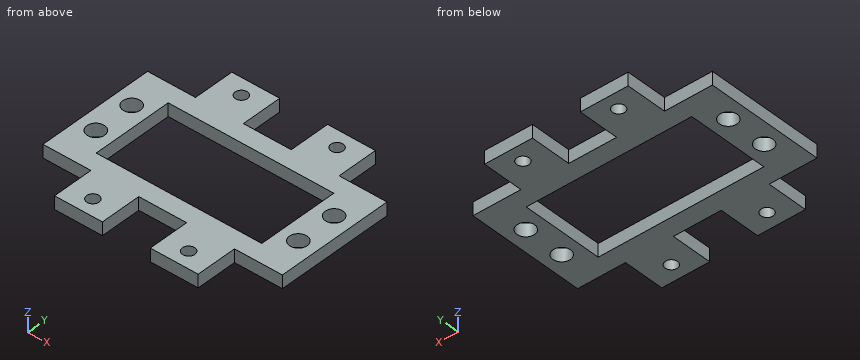
```python
from build123d import *

# Parameters (mm, degrees)
SKETCH2_R           = 2.15
SKETCH2_R_2         = 1.5
BOSS_EXTRUDE1_DEPTH = 3.175


with BuildPart() as part:
    # Sketch2 → Boss-Extrude1 (new body)
    with BuildSketch(Plane.XY):
        Polygon((23.312, 14.4), (29.14, 14.4), (29.14, 9.91), (8.98, 9.91), (8.98, 0), (0, 0), (0, 14.4), (11.656, 14.4), (11.656, 24.4), (23.312, 24.4), align=None)
        with Locations((4.49, 4.935)):
            Circle(SKETCH2_R, mode=Mode.SUBTRACT)
        with Locations((17.484, 20.43125)):
            Circle(SKETCH2_R_2, mode=Mode.SUBTRACT)
    boss_extrude1 = extrude(amount=BOSS_EXTRUDE1_DEPTH)

    # Mirror8: Boss-Extrude1 across plane
    add(boss_extrude1.mirror(Plane(origin=(8.98, 0, 3.175), x_dir=(0, 0, 1), z_dir=(0, 1, 0))))

    # Mirror10: part across plane


with BuildPart() as part_1:
    add(part.part)
    add(part.part.mirror(Plane(origin=(29.14, 9.91, 3.175), x_dir=(0, 0, 1), z_dir=(-1, 0, 0))))


solid = part_1.part
```
Read the model definition and answer for the solid it produces. Units are mm, in the model's axes. Round coordinates to 2 decimals unless told otherwise and drop trailing zeros. Write each loop counter-clockwise with the first axis right and the second up, starting at its lowest first coordinate (ties: lowest second). Pieces come first, ordered by that corner, then holes. Notation, with made-up numbers: (-4, 32) - (35, 32) arc R16 ccw to (35, 62) - close; hole circle Ø10 at (46.5, 42.25). An arc over 180 degrees is marked (long way). Use CSV: the item, a comma, the result in double quotes.
Q1. Find section C-C, the plane x = 53.79. Write down the section's boundary in (y, z) (3 decimals).
Values:
outline,"(-14.4, 0) - (-7.085, 0) - (-7.085, 3.175) - (-14.4, 3.175) - close; (-2.785, 0) - (2.785, 0) - (2.785, 3.175) - (-2.785, 3.175) - close; (7.085, 0) - (14.4, 0) - (14.4, 3.175) - (7.085, 3.175) - close"
Q2. Straight lines are drawn through the part: line 1 along X through (y, z) = (5, 0.45); line 2 along Y through (x, z) = (4.49, 1.6) (3 decimals); line 3 along Y through (x, z) = (37.5, 2). For each, find the intervals that lie inside material, in ascending order.
Values:
line 1,"x = 0 to 2.34, 6.64 to 8.98, 49.3 to 51.64, 55.94 to 58.28"
line 2,"y = -14.4 to -7.085, -2.785 to 2.785, 7.085 to 14.4"
line 3,"y = -24.4 to -9.91, 9.91 to 24.4"
Q3. Each of these flat-tipped pins is pushed along its axis until it touches: pin 1 Ø1.6 at (x, z) = (27.5, 2) entering from -Y; pin 2 Ø1 at (x, z) = (48.5, 2) entering from +Y. Where does it stop, or does it pass through?
Values:
pin 1,"stops at y = -14.4"
pin 2,"stops at y = 14.4"
Q4. Find section A-A, the plane x = 21. Write down the section's boundary in (y, z) (3 decimals), then the cut area to 3 significant figures.
Values:
outline,"(-24.4, 0) - (-9.91, 0) - (-9.91, 3.175) - (-24.4, 3.175) - close; (9.91, 0) - (24.4, 0) - (24.4, 3.175) - (9.91, 3.175) - close"
area,"92.0 mm²"
Q5. Find section B-B, the plane y = -8.5. Write down the section's boundary in (x, z) (3 decimals).
Values:
outline,"(0, 0) - (8.98, 0) - (8.98, 3.175) - (0, 3.175) - close; (49.3, 0) - (58.28, 0) - (58.28, 3.175) - (49.3, 3.175) - close"
Q6. Find section D-D, the plane z = 0.9. Count the separate pieces of the cut face and the enclosed holes in it, then the cut area to 3 significant figures.
Values:
separate pieces,"1"
enclosed holes,"9"
area,"1,260 mm²"
